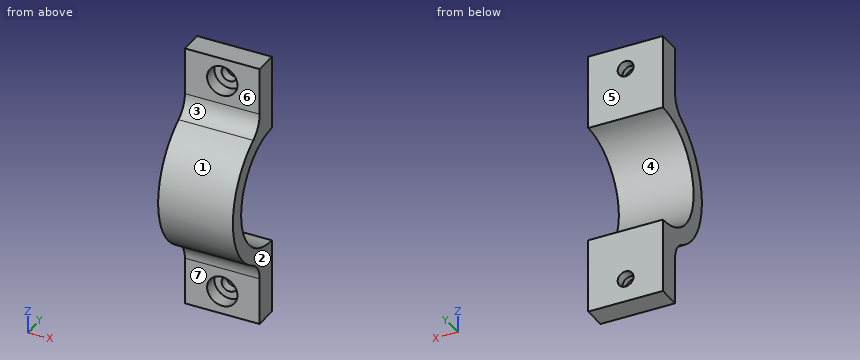
```python
from build123d import *

# Parameters (mm, degrees)
MOUNT_BOTTOM_DEPTH             = 8
FASTENING_FILET_BOTTOM_R       = 5
CBORE_FOR_M3_SHCS1_D           = 3.4
CBORE_FOR_M3_SHCS1_CBORE_D     = 6.5
CBORE_FOR_M3_SHCS1_CBORE_DEPTH = 3


with BuildPart() as part:
    # Sketch2 → Mount_Bottom (new, symmetric)
    with BuildSketch(Plane(origin=(0, 0, 0), x_dir=(0, 0, -1), z_dir=(1, 0, 0))):
        with BuildLine():
            Line((-12.6, 0), (-28.6, 0))
            Line((-28.6, 0), (-28.6, -5))
            Line((-28.6, -5), (-15.198684154, -5))
            ThreePointArc((-15.198684154, -5), (0, -16), (15.198684154, -5))
            Line((15.198684154, -5), (28.6, -5))
            Line((28.6, -5), (28.6, 0))
            Line((28.6, 0), (12.6, 0))
            ThreePointArc((12.6, 0), (0, -12.6), (-12.6, 0))
        make_face()
    extrude(amount=MOUNT_BOTTOM_DEPTH, both=True)

    # Fastening_Filet_Bottom
    fastening_filet_bottom_edges = [part.edges().sort_by_distance(p)[0] for p in [
        (0, -5, -15.198684154),
        (0, -5, 15.198684154),
    ]]
    fillet(fastening_filet_bottom_edges, radius=FASTENING_FILET_BOTTOM_R)

    # CBORE for M3 SHCS1 (through all)
    with Locations(Plane.XZ.offset(5)):
        with Locations((0, 23.6), (0, -23.6)):
            CounterBoreHole(CBORE_FOR_M3_SHCS1_D / 2, CBORE_FOR_M3_SHCS1_CBORE_D / 2, CBORE_FOR_M3_SHCS1_CBORE_DEPTH)


solid = part.part
```
Check sheet for the modelled part. Datum: model origin and axes. Units: mm. Face numbers are marked on the shaded views. A direction names the side the tool comes from. Give positions to 0.01 mm unless a question says otherwise; leave off trailing zeros. Order: outer loops, then holes, each group sorted by start corner. A loop starts at its lowest first (then second) coordinate and runs counter-clockwise, first axis right, second up. Notation, with made-up numbers: (80.5, 39) -> (131.5, 39) arc R31 ccw to (131.5, 66) -> close; hole circle Ø1 at (45, 40). An arc over 180 degrees is marked (long way). Return JSON: item names as keys, results as strings.
1. Set-up check for the marked faces 5, 6 and 7: record each of +Z, -Z, +X, -X, +Y, -Y from which the full face is reachable in a straight line by a thin tool's end or side.
From the geometry:
{"face 5": "+Z, -Z, +X, -X, +Y", "face 6": "+Z, +X, -X, -Y", "face 7": "-Z, +X, -X, -Y"}
2. Cross-section at D-D, the plane x = -6.5. Record the cut outline in (y, z).
From the geometry:
{"outline": "(-7.62, -14.07) arc R5 cw to (-5, -18.47) -> (-5, -28.6) -> (0, -28.6) -> (0, -12.6) arc R12.6 cw to (0, 12.6) -> (0, 28.6) -> (-5, 28.6) -> (-5, 18.47) arc R5 cw to (-7.62, 14.07) arc R16 ccw to start"}
3. Material ranges on probe 1 along Z at (x, y) = (0, -0.35); probe 2 along Z at (x, y) = (0, -3.35); probe 3 along X at (y, z) = (-4.5, -23.5), recorded low to high. Write a range as [from, to].
From the geometry:
{"probe 1": "[-28.6, -25.3], [-21.9, -12.6], [12.6, 21.9], [25.3, 28.6]", "probe 2": "[-28.6, -26.85], [-20.35, -12.15], [12.15, 20.35], [26.85, 28.6]", "probe 3": "[-8, -3.25], [3.25, 8]"}
4. Mould release check, pull along Z, two halves, no side actions. Record for the marked faces 1, 2, 3 and 4: +Z half, -Z half, draft (parallel to the pull), parting line (faces both ways), or undercut.
From the geometry:
{"face 1": "parting line", "face 2": "draft", "face 3": "+Z half", "face 4": "undercut"}
5. Cross-section at A-A, the plane y = -8.5. Record the cut outline in (x, z).
From the geometry:
{"outline": "(-8, -13.56) -> (8, -13.56) -> (8, -9.3) -> (-8, -9.3) -> close; (-8, 9.3) -> (8, 9.3) -> (8, 13.56) -> (-8, 13.56) -> close"}
6. Cross-section at B-B, the plane z = 23.6. Record the cut outline in (x, y), plus the area to 3 significant figures.
From the geometry:
{"outline": "(-8, -5) -> (-3.25, -5) -> (-3.25, -2) -> (-1.7, -2) -> (-1.7, 0) -> (-8, 0) -> close; (1.7, -2) -> (3.25, -2) -> (3.25, -5) -> (8, -5) -> (8, 0) -> (1.7, 0) -> close", "area": "53.7 mm^2"}
7. Cross-section at C-C, the plane x = 0.25. Record the cut outline in (y, z).
From the geometry:
{"outline": "(-7.62, -14.07) arc R5 cw to (-5, -18.47) -> (-5, -20.36) -> (-2, -20.36) -> (-2, -21.92) -> (0, -21.92) -> (0, -12.6) arc R12.6 cw to (0, 12.6) -> (0, 21.92) -> (-2, 21.92) -> (-2, 20.36) -> (-5, 20.36) -> (-5, 18.47) arc R5 cw to (-7.62, 14.07) arc R16 ccw to start; (-5, -28.6) -> (0, -28.6) -> (0, -25.28) -> (-2, -25.28) -> (-2, -26.84) -> (-5, -26.84) -> close; (-5, 26.84) -> (-2, 26.84) -> (-2, 25.28) -> (0, 25.28) -> (0, 28.6) -> (-5, 28.6) -> close"}
8. Go/stop test with flat-tipped pins: P1, Ø1, axis at x = 5, y = -7, coming from the +Z side; P2, Ø7.5, axis at x = 0, z = 23.6, coming from the -Y side; P3, Ø2, axis at x = 6.5, y = -8, coming from the -Z side. Record where each tip stops, or that it passes through.
From the geometry:
{"P1": "z = 14.9", "P2": "y = -5", "P3": "z = -14.47"}
